Here's how the part is built. I have some questions about the finished solid (model axes, mm). Face numbers are marked on the shaded views. Round coordinates to 2 decimals unless told otherwise and drop trailing zeros. Order: outer loops, then holes, each group sorted by start corner. A loop starts at its lowest first (then second) coordinate and runs counter-clockwise, first axis right, second up. Notation, with made-up numbers: (55.25, 72.5) - (77.25, 72.5) arc R10 ccw to (77.25, 87.5) - close; hole circle Ø11 at (12.5, 63.5). An arc over 180 degrees is marked (long way). Answer as a JSON object with one key per item and string values.
```python
from build123d import *

# Parameters (mm, degrees)
SKETCH1_W           = 40.5
SKETCH1_H           = 16
SKETCH1_R           = 1.35
BOSS_EXTRUDE1_DEPTH = 12
BOSS_EXTRUDE2_START = 2
BOSS_EXTRUDE2_DEPTH = 10
BOSS_EXTRUDE3_DEPTH = 40.5
SKETCH4_R           = 2
CUT_EXTRUDE3_DEPTH  = 40.502331785
CUT_EXTRUDE4_START  = -3
SKETCH4_5_R         = 3.5
SKETCH4_5_R_2       = 2
CUT_EXTRUDE4_DEPTH  = 37.502331785
CHAMFER2_SIZE       = 1
FILLET2_R           = 5


with BuildPart() as part:
    # Sketch1 → Boss-Extrude1 (new body)
    with BuildSketch(Plane(origin=(0, 0, 0), x_dir=(1, 0, 0), z_dir=(0, 1, 0))):
        Rectangle(SKETCH1_W, SKETCH1_H)
        with Locations(Location((-17.25, 5, 0), (0, 0, 270))):
            Circle(SKETCH1_R, mode=Mode.SUBTRACT)
        with BuildLine():
            Line((-14.421572875, 6), (-1.078427125, 6))
            ThreePointArc((-1.078427125, 6), (1.75, 2), (4.578427125, 6))
            Line((4.578427125, 6), (18.25, 6))
            Line((18.25, 6), (18.25, -6))
            Line((18.25, -6), (-18.25, -6))
            Line((-18.25, -6), (-18.25, 2.171572875))
            ThreePointArc((-18.25, 2.171572875), (-15.128679656, 2.878679656), (-14.421572875, 6))
        make_face(mode=Mode.SUBTRACT)
        with Locations(Location((1.75, 5, 0), (0, 0, 270))):
            Circle(SKETCH1_R, mode=Mode.SUBTRACT)
    extrude(amount=BOSS_EXTRUDE1_DEPTH)

    # Sketch1<3> → Boss-Extrude2 (add)
    with BuildSketch(Plane(origin=(0, 0, 0), x_dir=(1, 0, 0), z_dir=(0, 1, 0)).offset(BOSS_EXTRUDE2_START)):
        with BuildLine():
            ThreePointArc((-14.25, 5), (-15.517949192, 2.550510257), (-18.25, 2.171572875))
            Line((-18.25, 2.171572875), (-18.25, -6))
            Line((-18.25, -6), (18.25, -6))
            Line((18.25, -6), (18.25, 6))
            Line((18.25, 6), (4.578427125, 6))
            ThreePointArc((4.578427125, 6), (4.706795679, 5.507305936), (4.75, 5))
            ThreePointArc((4.75, 5), (1.242694064, 2.043204321), (-1.078427125, 6))
            Line((-1.078427125, 6), (-14.421572875, 6))
            ThreePointArc((-14.421572875, 6), (-14.293204321, 5.507305936), (-14.25, 5))
        make_face()
    extrude(amount=BOSS_EXTRUDE2_DEPTH)

    # Sketch3 → Boss-Extrude3 (add)
    with BuildSketch(Plane.ZY.offset(20.25)):
        Polygon((8, 0), (17.899494937, -9.899494937), (32.04163056, 4.242640687), (24.284271247, 12), (8, 12), align=None)
    extrude(amount=-BOSS_EXTRUDE3_DEPTH)

    # Sketch4 → Cut-Extrude3 (cut, through all)
    with BuildSketch(Plane(origin=(0, -13.899494937, 13.899494937), x_dir=(1, 0, 0), z_dir=(0, -0.7071067811865437, 0.7071067811865513))):
        with Locations(Location((-10, 15.656854249, 0), (0, 0, 270))):
            Circle(SKETCH4_R)
        with Locations(Location((10, 15.656854249, 0), (0, 0, 270))):
            Circle(SKETCH4_R)
    extrude(amount=-CUT_EXTRUDE3_DEPTH, mode=Mode.SUBTRACT)

    # Sketch4<5> → Cut-Extrude4 (cut, through all)
    # profile 1 of 2: a face of its own
    with BuildSketch(Plane(origin=(0, -13.899494937, 13.899494937), x_dir=(1, 0, 0), z_dir=(0, -0.7071067811865437, 0.7071067811865513)).offset(CUT_EXTRUDE4_START)):
        with Locations(Location((10, 15.656854249, 0), (0, 0, 270))):
            Circle(SKETCH4_5_R)
        with Locations(Location((10, 15.656854249, 0), (0, 0, 270))):
            Circle(SKETCH4_5_R_2, mode=Mode.SUBTRACT)
    # profile 2 of 2: a face of its own
    with BuildSketch(Plane(origin=(0, -13.899494937, 13.899494937), x_dir=(1, 0, 0), z_dir=(0, -0.7071067811865437, 0.7071067811865513)).offset(CUT_EXTRUDE4_START)):
        with Locations(Location((-10, 15.656854249, 0), (0, 0, 90))):
            Circle(SKETCH4_5_R)
        with Locations(Location((-10, 15.656854249, 0), (0, 0, 270))):
            Circle(SKETCH4_5_R_2, mode=Mode.SUBTRACT)
    extrude(amount=-CUT_EXTRUDE4_DEPTH, mode=Mode.SUBTRACT)

    # Chamfer2
    chamfer2_edges = [part.edges().sort_by_distance(p)[0] for p in [
        (-10, 0.707106781, 24.263455967),
        (10, 0.707106781, 24.263455967),
    ]]
    chamfer(chamfer2_edges, length=CHAMFER2_SIZE)

    # Fillet2
    # the kernel refuses this fillet: 5 mm, written as the material it takes off along each edge
    with BuildSketch(Plane(origin=(15.25, 7, 22.213203436), x_dir=(0, 0.7071067811865516, 0.7071067811865435), z_dir=(1, 0, 0))) as fillet2_piece_1_section:
        Polygon((0, 0), (FILLET2_R, 0), (FILLET2_R, -FILLET2_R * 0.414213562373), (FILLET2_R * 0.707106781187, -FILLET2_R * 0.707106781187), align=None)
    fillet2_piece_1 = extrude(amount=FILLET2_R, mode=Mode.PRIVATE)
    fillet2_piece_1 = fillet2_piece_1 - Plane(origin=(15.25, 7, 22.213203436), x_dir=(0, -0.9238795325112877, -0.3826834323650871), z_dir=(1, 0, 0)) * Sphere(FILLET2_R, mode=Mode.PRIVATE)
    add(fillet2_piece_1, mode=Mode.SUBTRACT)
    with BuildSketch(Plane(origin=(-15.25, 7, 22.213203436), x_dir=(0, 0.7071067811865516, 0.7071067811865435), z_dir=(-1, 0, 0))) as fillet2_piece_2_section:
        Polygon((0, 0), (FILLET2_R, 0), (FILLET2_R, FILLET2_R * 0.414213562373), (FILLET2_R * 0.707106781187, FILLET2_R * 0.707106781187), align=None)
    fillet2_piece_2 = extrude(amount=FILLET2_R, mode=Mode.PRIVATE)
    fillet2_piece_2 = fillet2_piece_2 - Plane(origin=(-15.25, 7, 22.213203436), x_dir=(0, -0.9238795325112877, -0.3826834323650871), z_dir=(-1, 0, 0)) * Sphere(FILLET2_R, mode=Mode.PRIVATE)
    add(fillet2_piece_2, mode=Mode.SUBTRACT)
    with BuildSketch(Plane(origin=(20.25, -4.596194078, 40.880465325), x_dir=(0, -0.7071067811865516, -0.7071067811865435), z_dir=(0, 0.7071067811865435, -0.7071067811865516))) as fillet2_piece_3:
        with BuildLine():
            CenterArc((FILLET2_R, FILLET2_R), FILLET2_R, 180, 90)
            Line((0, FILLET2_R), (0, 0))
            Line((0, 0), (FILLET2_R, 0))
        make_face()
    extrude(amount=21.399494937, mode=Mode.SUBTRACT)
    with BuildSketch(Plane(origin=(-20.25, -4.596194078, 40.880465325), x_dir=(0, -0.7071067811865516, -0.7071067811865435), z_dir=(0, 0.7071067811865435, -0.7071067811865516))) as fillet2_piece_4:
        with BuildLine():
            CenterArc((FILLET2_R, -FILLET2_R), FILLET2_R, 90, 90)
            Line((0, -FILLET2_R), (0, 0))
            Line((0, 0), (FILLET2_R, 0))
        make_face()
    extrude(amount=21.399494937, mode=Mode.SUBTRACT)
    with BuildSketch(Plane(origin=(20.25, 12, -20.5), x_dir=(0, -1, 0), z_dir=(0, 0, 1)), Plane(origin=(-20.25, 12, 22.213203436), x_dir=(0, -1, 0), z_dir=(0, 0, -1))) as fillet2_piece_5:
        with BuildLine():
            CenterArc((FILLET2_R, -FILLET2_R), FILLET2_R, 90, 90)
            Line((0, -FILLET2_R), (0, 0))
            Line((0, 0), (FILLET2_R, 0))
        make_face()
    extrude(amount=42.713203436, mode=Mode.SUBTRACT)
    with BuildSketch(Plane(origin=(-15.25, 12, 24.284271247), x_dir=(0, -0.7071067811865432, 0.7071067811865519), z_dir=(1, 0, 0))) as fillet2_piece_6:
        with BuildLine():
            CenterArc((FILLET2_R * 0.414213562373, FILLET2_R), FILLET2_R, 225, 45)
            Line((-FILLET2_R * 0.292893218813, FILLET2_R * 0.292893218813), (0, 0))
            Line((0, 0), (FILLET2_R * 0.414213562373, 0))
        make_face()
    extrude(amount=30.5, mode=Mode.SUBTRACT)
    with BuildSketch(Plane(origin=(32.75, 12, -8), x_dir=(0, -1, 0), z_dir=(-1, 0, 0))) as fillet2_piece_7:
        with BuildLine():
            CenterArc((FILLET2_R, FILLET2_R), FILLET2_R, 180, 90)
            Line((0, FILLET2_R), (0, 0))
            Line((0, 0), (FILLET2_R, 0))
        make_face()
    extrude(amount=65.5, mode=Mode.SUBTRACT)


solid = part.part
```
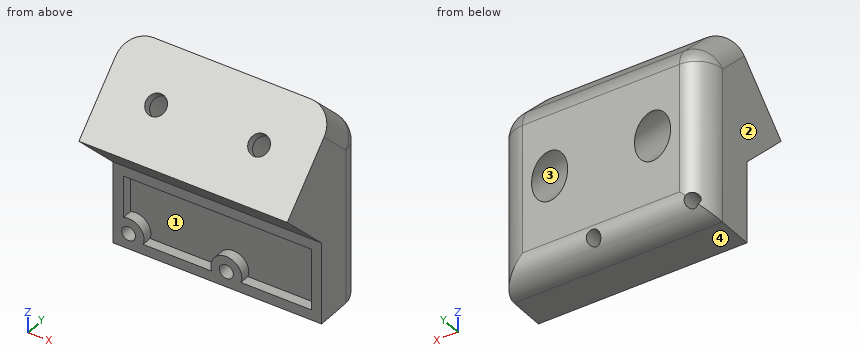
1. Imagine slicing it at C-C (z = 17). Give the number of separate pieces and of enclosed holes in the cut face, plus the area to 3 significant figures.
Responses:
{"separate pieces": "1", "enclosed holes": "2", "area": "731 mm2"}
2. Imagine slicing it at D-D (y = -6.25). List the corners of the cut face in (x, z) for me, plus the area to 3 significant figures.
Responses:
{"outline": "(-20.25, 14.25) - (20.25, 14.25) - (20.25, 21.55) - (-20.25, 21.55) - close", "area": "296 mm2"}
3. Imagine slicing it at B-B (z = -5). List the corners of the cut face in (x, y) for me, plus the area to 3 significant figures.
Responses:
{"outline": "(-20.25, 0) - (-18.6, 0) - (-18.6, 10.71) arc R5 ccw to (-20.25, 7) - close; (-15.9, 0) - (-14.25, 0) - (-14.25, 2) - (-1.25, 2) - (-1.25, 0) - (0.4, 0) - (0.4, 11.58) - (-15.9, 11.58) - close; (3.1, 0) - (4.75, 0) - (4.75, 2) - (18.25, 2) - (18.25, 0) - (20.25, 0) - (20.25, 7) arc R5 ccw to (17.25, 11.58) - (3.1, 11.58) - close", "area": "346 mm2"}
4. If I drill on L1, parallel to X at y = 7, z = -5; L2, parallel to Y at x = -14.5, z = 15; L3, parallel to Z at x = -17.25, y = 4, over which ranges is the centre line in solid material (lowest first)? Write a range as [from, to].
Responses:
{"L1": "[-20.25, -18.6], [-15.9, 0.4], [3.1, 20.25]", "L2": "[-7, 12]", "L3": "[-8, -6.35], [-3.65, 31.69]"}
5. For P1, Ø2, axis at x = 1.75, z = -5, coming from the -Y side; P2, Ø6, axis at x = 16, z = 14.5, coming from the -Y side; P3, Ø1, axis at x = 14, y = 1, coming from the +Z side; P4, Ø3.5, axis at x = -17.25, z = -5, coming from the +Y side, each with a flat end and sliding along its axis, tell me the tip position at first contact or that it passes through.
Responses:
{"P1": "through", "P2": "y = -9.5", "P3": "z = 29.3", "P4": "y = 11.94"}
6. Imagine slicing it at A-A (x = 2.5). List the corners of the cut face in (y, z) for me.
Responses:
{"outline": "(-9.9, 17.9) - (0, 8) - (0, 6) - (2, 6) - (2, -2.1) - (0, -2.1) - (0, -3.88) - (11.92, -3.88) arc R5 ccw to (12, -3) - (12, 22.21) arc R5 ccw to (10.54, 25.75) - (4.24, 32.04) - close; (0, -8) - (7, -8) arc R5 ccw to (10.91, -6.12) - (0, -6.12) - close"}
7. Thinking about a two-plate mould opening in Z: for the marked faces 1, 2, 3 and 4, which applies, pulls with the +Z half, pulls with the -Z half, needs draft (parallel to the pull), parting line crosses it, or undercut?
Responses:
{"face 1": "undercut", "face 2": "needs draft", "face 3": "undercut", "face 4": "pulls with the -Z half"}
